Read the model definition and answer for the solid it produces. Units are mm, in the model's axes. A direction names the side the tool comes from. Round coordinates to 2 decimals unless told otherwise and drop trailing zeros. Write each loop counter-clockwise with the first axis right and the second up, starting at its lowest first coordinate (ties: lowest second). Pieces come first, ordered by that corner, then holes. Notation, with made-up numbers: (30, 60.25) -> (80, 60.25) arc R9 ccw to (80, 64.25) -> close; hole circle Ø6 at (36.5, 84). An arc over 180 degrees is marked (long way). Return JSON: item names as keys, results as strings.
from build123d import *

# Parameters (mm, degrees)
F1_DEPTH = 14
F2_DEPTH = 7


with BuildPart() as f1:
    # F0 (on Top) → F1 (new body)
    with BuildSketch(Plane.XY):
        Polygon((-12.239826, 0.433735), (-6.119913, -10.166265), (6.119913, -10.166265), (12.239826, 0.433735), (6.119913, 11.033735), (-6.119913, 11.033735), align=None)
        Polygon((10.392305, 0.433735), (5.196152, -8.566265), (-5.196152, -8.566265), (-10.392305, 0.433735), (-5.196152, 9.433735), (5.196152, 9.433735), align=None, mode=Mode.SUBTRACT)
        Polygon((-5.196152, -8.566265), (5.196152, -8.566265), (10.392305, 0.433735), (5.196152, 9.433735), (-5.196152, 9.433735), (-10.392305, 0.433735), align=None)
    extrude(amount=-F1_DEPTH)

    # F0 (on Top) → F2 (join)
    with BuildSketch(Plane.XY):
        Polygon((-12.239826, 0.433735), (-6.119913, -10.166265), (6.119913, -10.166265), (12.239826, 0.433735), (6.119913, 11.033735), (-6.119913, 11.033735), align=None)
        Polygon((10.392305, 0.433735), (5.196152, -8.566265), (-5.196152, -8.566265), (-10.392305, 0.433735), (-5.196152, 9.433735), (5.196152, 9.433735), align=None, mode=Mode.SUBTRACT)
    extrude(amount=F2_DEPTH)


solid = f1.part
Item 1: Section C-C (y = -2) is taken. Give the vertices of the cut face in (x, z).
Worked answers:
{"outline": "(-10.83, -14) -> (10.83, -14) -> (10.83, 7) -> (8.99, 7) -> (8.99, 0) -> (-8.99, 0) -> (-8.99, 7) -> (-10.83, 7) -> close"}
Item 2: A tool of negligible diameter and unlimited length cuts with its end or side. For faces 1 (the flat face through (-7.83, 4.87, 3.45)), 2 (the flat face through (7, -6, 7)), from which of +Z, -Z, +X, -X, +Y, -Y can it reach the whole face along a straight path? Write none if from no direction.
Worked answers:
{"face 1": "+Z", "face 2": "+Z, +X, -X, +Y, -Y"}
Item 3: Section D-D (z = -11.75) is taken. Give the vertices of the cut face in (x, y).
Worked answers:
{"outline": "(-12.24, 0.43) -> (-6.12, -10.17) -> (6.12, -10.17) -> (12.24, 0.43) -> (6.12, 11.03) -> (-6.12, 11.03) -> close"}
Item 4: Straight lines are drawn through the part: L1, parallel to Y at x = -0.25, z = 4; L2, parallel to Z at x = -4.25, y = 7; L3, parallel to Y at x = 5.25, z = 2.25. For each, find the intervals that lie inside material, in ascending order. Write a range as [from, to].
Worked answers:
{"L1": "y = [-10.17, -8.57], [9.43, 11.03]", "L2": "z = [-14, 0]", "L3": "y = [-10.17, -8.47], [9.34, 11.03]"}
Item 5: For a pull along X with two mould halves and no side action, classify faces 3 (the flat face through (9.137, -4.94, -3.647)), 4 (the flat face through (-9.223, -4.792, -3.647)), 5 (the flat face through (0, 9.434, 3)), 6 (the flat face through (0, 1, -14)) as released by +X, released by -X, zero draft, split by the parting line, or undercut.
Worked answers:
{"face 3": "released by +X", "face 4": "released by -X", "face 5": "undercut", "face 6": "zero draft"}
Item 6: Section B-B (x = 1.75) is taken. Give the vertices of the cut face in (y, z).
Worked answers:
{"outline": "(-10.17, -14) -> (11.03, -14) -> (11.03, 7) -> (9.43, 7) -> (9.43, 0) -> (-8.57, 0) -> (-8.57, 7) -> (-10.17, 7) -> close"}
Item 7: Section A-A (z = 0.75) is taken. Give the vertices of the cut face in (x, y), then the cut area to 3 significant figures.
Worked answers:
{"outline": "(-12.24, 0.43) -> (-6.12, -10.17) -> (6.12, -10.17) -> (12.24, 0.43) -> (6.12, 11.03) -> (-6.12, 11.03) -> close; hole (-10.39, 0.43) -> (-5.2, -8.57) -> (5.2, -8.57) -> (10.39, 0.43) -> (5.2, 9.43) -> (-5.2, 9.43) -> close", "area": "109 mm2"}
Item 8: Flat-ended cylindrical pins translate along their axes: pin 1 (10 mm diameter, centred on y = -0.5, z = -4.5, fed in from -X); pin 2 (10 mm diameter, centred on x = -1, y = -1.5, fed in from +Z); pin 3 (8 mm diameter, centred on y = 7, z = 1.5, fed in from +X); pin 4 (5 mm diameter, centred on x = -7, z = 3, fed in from -Y). Find the tip coordinate at first contact, or state that the pin passes through.
Worked answers:
{"pin 1": "stops at x = -12.24", "pin 2": "stops at z = 0", "pin 3": "stops at x = 10.76", "pin 4": "stops at y = -10.17"}
